from build123d import *

# Parameters (mm, degrees)
EXTRUDE_1_DEPTH     = 5
SKETCH_2_R          = 2.2
CUT_EXTRUDE_1_DEPTH = 14.747727085
EXTRUDE_START       = -5.8
EXTRUDE_2_DEPTH     = 5.8
FILLET_1_R          = 1


with BuildPart() as part:
    # 草图1 → 凸台-拉伸1 (new, symmetric)
    with BuildSketch(Plane.XY):
        with BuildLine():
            Line((2.1, -2.1), (10, -2.1))
            Line((10, -2.1), (10, 5.9))
            Line((10, 5.9), (-10, 5.9))
            Line((-10, 5.9), (-10, -2.1))
            Line((-10, -2.1), (-2.1, -2.1))
            Line((-2.1, -2.1), (-2.1, 0))
            ThreePointArc((-2.1, 0), (0, 2.1), (2.1, 0))
            Line((2.1, 0), (2.1, -2.1))
        make_face()
    extrude(amount=EXTRUDE_1_DEPTH, both=True)

    # 草图2 → 切除-拉伸1 (cut, through all)
    with BuildSketch(Plane(origin=(0, 5.9, 0), x_dir=(1, 0, 0), z_dir=(0, 1, 0))):
        with Locations(Location((-6, 0, 0), (0, 0, 270))):
            Circle(SKETCH_2_R)
        with Locations(Location((6, 0, 0), (0, 0, 270))):
            Circle(SKETCH_2_R)
    extrude(amount=-CUT_EXTRUDE_1_DEPTH, mode=Mode.SUBTRACT)

    # 草图3 → 凸台-拉伸2 (add)
    with BuildSketch(Plane(origin=(0, 0, -5), x_dir=(-1, 0, 0), z_dir=(0, 0, -1)).offset(EXTRUDE_START)):
        with BuildLine():
            Line((2.1, -2.1), (2.1, 0))
            ThreePointArc((2.1, 0), (0, 2.1), (-2.1, 0))
            Line((-2.1, 0), (-2.1, -2.1))
            Line((-2.1, -2.1), (2.1, -2.1))
        make_face()
    extrude(amount=EXTRUDE_2_DEPTH)

    # 圆角1
    fillet_1_edges = [part.edges().sort_by_distance(p)[0] for p in [
        (-10, 1.9, -5),
        (10, 1.9, 5),
        (-10, 1.9, 5),
        (10, 1.9, -5),
    ]]
    fillet(fillet_1_edges, radius=FILLET_1_R)


solid = part.part
Design review of the part built by this model. Coordinates are the model's own, in mm. A direction names the side the tool comes from. Round coordinates to 2 decimals unless told otherwise and drop trailing zeros. Write each loop counter-clockwise with the first axis right and the second up, starting at its lowest first coordinate (ties: lowest second). Pieces come first, ordered by that corner, then holes. Notation, with made-up numbers: (-13.75, 8.25) -> (32.25, 8.25) arc R34 ccw to (32.25, 39.25) -> close; hole circle Ø2 at (24, 82.5). An arc over 180 degrees is marked (long way). One line per item, written item: value. Start each with the question number.
Q1. Add section C-C (z = 1). Give the boundary of the cut face in (x, y).
Q2. To check wall thickness, follow probe 1 along X at (y, z) = (3.75, 0); probe 2 along X at (y, z) = (-0.75, 1.75); probe 3 along X at (y, z) = (5.25, -0.5). State the ranges of each line that lie inside material, in increasing order.
Q3. The part is to be moulded in two halves that separate along Z. For faces 1 (the face through (0, 3, 5)), 2 (the face through (0, 5.9, 0)), 3 (the face through (-8.148, 1.956, -0.477)), say which applies: pulls with the +Z half, pulls with the -Z half, needs draft (parallel to the pull), parting line crosses it, or undercut.
Q4. Add section D-D (x = 0). Give the boundary of the cut face in (y, z).
Q5. Add section A-A (x = 6). Give the boundary of the cut face in (y, z), then the cut area to 3 significant figures.
Q6. Tool access review of faces 4 (the face through (-2.1, -1, 3)), 5 (the face through (0, -2.1, 0)): name each direction out of +Z, -Z, +X, -X, +Y, -Y from which nothing blocks a thin tool from reaching the whole face with its end or side.
Q7. Add section B-B (y = -1.25). Give the boundary of the cut face in (x, z), then the cut area to 3 significant figures.
Response:
1. outline: (-10, -2.1) -> (-7.96, -2.1) -> (-7.96, 5.9) -> (-10, 5.9) -> close; (-4.04, -2.1) -> (-2.1, -2.1) -> (-2.1, 0) arc R2.1 cw to (2.1, 0) -> (2.1, -2.1) -> (4.04, -2.1) -> (4.04, 5.9) -> (-4.04, 5.9) -> close; (7.96, -2.1) -> (10, -2.1) -> (10, 5.9) -> (7.96, 5.9) -> close
2. probe 1: x = -10 to -8.2, -3.8 to 3.8, 8.2 to 10
2. probe 2: x = -10 to -7.33, -4.67 to -2.1, 2.1 to 4.67, 7.33 to 10
2. probe 3: x = -10 to -8.14, -3.86 to 3.86, 8.14 to 10
3. face 1: pulls with the +Z half
3. face 2: needs draft
3. face 3: undercut
4. outline: (-2.1, -5) -> (5.9, -5) -> (5.9, 5) -> (2.1, 5) -> (2.1, 0.8) -> (-2.1, 0.8) -> close
5. outline: (-2.1, -5) -> (5.9, -5) -> (5.9, -2.2) -> (-2.1, -2.2) -> close; (-2.1, 2.2) -> (5.9, 2.2) -> (5.9, 5) -> (-2.1, 5) -> close
5. area: 44.8 mm^2
6. face 4: +Z, -Y
6. face 5: +Z, -Z, +X, -X, -Y
7. outline: (-10, -4) arc R1 ccw to (-9, -5) -> (9, -5) arc R1 ccw to (10, -4) -> (10, 4) arc R1 ccw to (9, 5) -> (2.1, 5) -> (2.1, 0.8) -> (-2.1, 0.8) -> (-2.1, 5) -> (-9, 5) arc R1 ccw to (-10, 4) -> close; hole circle Ø4.4 at (-6, 0); hole circle Ø4.4 at (6, 0)
7. area: 151 mm^2
